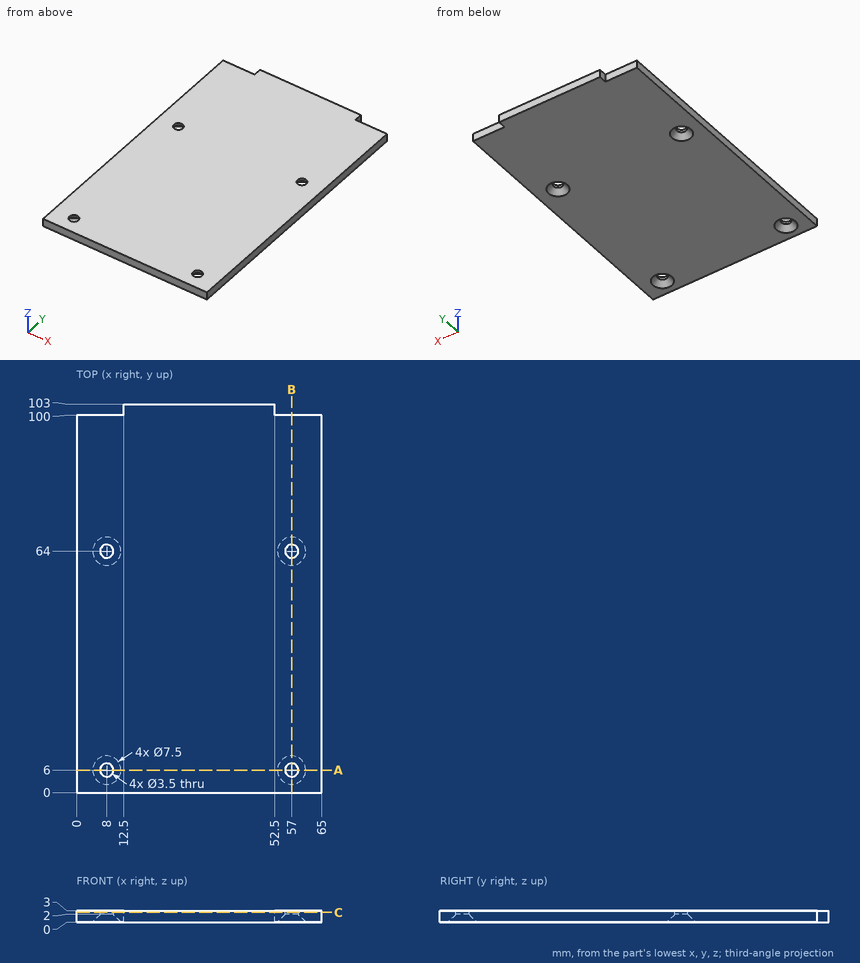
Here's the drawing with two shaded views (mm, measured from the low corner). I have some questions. Coordinates: 2 decimals unless noted, no trailing zeros. Loops run counter-clockwise (first coordinate to the right, second up) from the corner with the lowest first, then second, coordinate; pieces in that order, holes last. Notation, with made-up numbers: (32.25, 84) - (77.25, 84) arc R21 cw to (77.25, 95) - close; hole circle Ø9 at (23.25, -35.75). An arc over 180 degrees is marked (long way). Answer as CSV lines item,"result". Start each with the question number.
1) For pin 1 (0.9 mm diameter, centred on y = 101.5, z = 1, fed in from -X); pin 2 (3 mm diameter, centred on x = 8, y = 64, fed in from -Z) (3 decimals); pin 3 (1.5 mm diameter, centred on x = 58.5, z = 1, fed in from +Y), each with a flat end and sliding along its axis, tell me the tip position at first contact or that it passes through.
2) Suppose I cut it at B-B (x = 57). Please give me the cut outline in (y, z), plus the area to 3 significant figures.
3) I need wall thicknesses on line 1 (X direction, y = 64, z = 2.5); line 2 (Y direction, x = 8, z = 2.55); line 3 (Y direction, x = 10.5, z = 2.15). Which ranges of each line are inside material? Lowest first, please. Write a range as from..to.
4) Suppose I cut it at A-A (y = 6). Please give me the cut outline in (x, z), plus the area to 3 significant figures.
5) Suppose I cut it at C-C (z = 2.55). Please give me the cut outline in (x, y).
Check result:
1,pin 1,"stops at x = 12.5"
1,pin 2,"passes through"
1,pin 3,"stops at y = 100"
2,outline,"(0, 0) - (2.25, 0) - (4.25, 2) - (4.25, 3) - (0, 3) - close; (7.75, 2) - (9.75, 0) - (60.25, 0) - (62.25, 2) - (62.25, 3) - (7.75, 3) - close; (65.75, 2) - (67.75, 0) - (100, 0) - (100, 3) - (65.75, 3) - close"
2,area,"271 mm²"
3,line 1,"x = 0..6.25, 9.75..55.25, 58.75..65"
3,line 2,"y = 0..4.25, 7.75..62.25, 65.75..100"
3,line 3,"y = 0..100"
4,outline,"(0, 0) - (4.25, 0) - (6.25, 2) - (6.25, 3) - (0, 3) - close; (9.75, 2) - (11.75, 0) - (53.25, 0) - (55.25, 2) - (55.25, 3) - (9.75, 3) - close; (58.75, 2) - (60.75, 0) - (65, 0) - (65, 3) - (58.75, 3) - close"
4,area,"166 mm²"
5,outline,"(0, 0) - (65, 0) - (65, 100) - (52.5, 100) - (52.5, 103) - (12.5, 103) - (12.5, 100) - (0, 100) - close; hole circle Ø3.5 at (8, 6); hole circle Ø3.5 at (8, 64); hole circle Ø3.5 at (57, 6); hole circle Ø3.5 at (57, 64)"
